Design review of the part built by this model. Coordinates are the model's own, in mm. A direction names the side the tool comes from. Coordinates: 2 decimals unless noted, no trailing zeros. Order: outer loops, then holes, each group sorted by start corner. A loop starts at its lowest first (then second) coordinate and runs counter-clockwise, first axis right, second up. Notation, with made-up numbers: (82.5, 78) -> (121.5, 78) arc R33 cw to (121.5, 108) -> close; hole circle Ø2 at (2.5, 51). An arc over 180 degrees is marked (long way). Use a Markdown table: item, result. Add a question column.
Q1. Add section C-C (x = -0.5). State the section outline as (y, z) points, then the cut area to 3 significant figures.
Q2. Wall thickness on probe 1 along X at (y, z) = (20, 1.1); probe 2 along X at (y, z) = (11.5, 0.85); probe 3 along X at (y, z) = (17, 5.6): over which ranges is each line inside the solid? List them lowest first.
Q3. Insertion check: pin 1 (3 mm diameter, centred on y = 14, z = 3, fed in from -X); pin 2 (1.8 mm diameter, centred on y = -2, z = 2, fed in from +X); pin 3 (0.9 mm diameter, centred on x = 11.5, z = 2.5, fed in from -Y). Each pin has a flat end and moves straight along its axis. Give the tip position at first contact, or say it passes through.
Q4. Machinability: for faces 1 (the face through (10, 15, 3)), 2 (the face through (7.21, 20.62, 3.04)), 3 (the face through (11, 0, 3)), 4 (the face through (-2, 0, 3)), 5 (the face through (13, 1, 3)), which of the approach directions +Z, -Z, +X, -X, +Y, -Y give a long, thin tool a straight path to every point of the face, cutting with its end or side? Answer none if there is none.
Q5. The part is to be moulded in two halves that separate along X. For faces 6 (the face through (4.96, 15.25, 3.04)), 7 (the face through (1, 25, 3)), 8 (the face through (0, 15, 3)), say which applies: pulls with the +X half, pulls with the -X half, needs draft (parallel to the pull), parting line crosses it, or undercut.
Q6. Add section B-B (y = -3). State the section outline as (x, z) points.
Autodesk Inventor part; units mm, degrees
ref_plane "YZ Plane" through (0, 0, 0) normal (1, 0, 0) x (0, 1, 0)
ref_plane "XZ Plane" through (0, 0, 0) normal (0, 1, 0) x (-1, 0, 0)
ref_plane "XY Plane" through (0, 0, 0) normal (0, 0, 1) x (1, 0, 0)
sketch "Sketch1" plane through (0, 0, 0) normal (0, 0, 1) x (1, 0, 0)
  line L0 (0, -6) -> (0, 0)
  line L1 (-9, 0) -> (0, 0)
  line L2 (0, -6) -> (-9, -6)
  line L3 (0, 0) -> (10, 0)
  line L4 (0, 0) -> (0, -6)
  line L5 (10, -6) -> (0, -6)
  line L6 (10, 0) -> (10, -6)
  line L7 (0, -6) -> (-9, -6)
  line L8 (-9, 0) -> (0, 0)
  line L9 (0, -6) -> (10, -6)
  line L10 (10, -6) -> (10, 0)
  line L11 (10, 0) -> (0, 0)
  line L12 (0, 0) -> (0, -6)
  line L13 (-3, 0) -> (13, 0)
  line L14 (13, 0) -> (13, 2)
  line L15 (13, 2) -> (-3, 2)
  line L16 (-3, 2) -> (-3, 0)
  line L17 (-9, -6) -> (-9, 0)
  line L18 (-9, -6) -> (-9, 0)
  line L19 (0, -6) -> (0, 0)
  point P0 (5, 2)
  point P1 (5, 0)
  dimension "d0" = 16
  dimension "d2" = 2
extrude "Extrusion1" add sketch "Sketch1" along normal blind 6 contours L0 L3 L6 L5 | L1 L16 L15 L14 L13 L3
sketch "Sketch2" plane through (0, 0, 6) normal (0, 0, 1) x (1, 0, 0)
  line L0 (0, 0) -> (0, -6)
  line L1 (0, -6) -> (10, -6)
  line L2 (10, -6) -> (10, 0)
  line L3 (13, 2) -> (-3, 2)
  line L4 (0, 2) -> (10, 2)
  line L5 (10, 2) -> (10, 25)
  line L6 (10, 25) -> (0, 25)
  line L7 (0, 25) -> (0, 2)
  dimension "d6" = 31
  dimension "d21" = 10
extrude "Extrusion2" add sketch "Sketch2" against normal blind 6
chamfer "Chamfer1" distance 3 angle 45 2 edges at (0, 2, 3) (10, 2, 3)
sketch "Sketch3" plane through (0, 0, 6) normal (0, 0, 1) x (1, 0, 0)
  line L0 (10, 5) -> (10, 25)
  line L1 (10, 25) -> (0, 25)
  line L2 (0, 25) -> (0, 5)
  line L3 (2.25, 25) -> (7.75, 25)
  line L4 (7.75, 25) -> (7.75, 17) construction
  line L5 (7.75, 17) -> (2.25, 17) construction
  line L6 (2.25, 17) -> (2.25, 25) construction
  circle A0 centre (5, 17) radius 1.75
  line L7 (-3, 0) -> (0, 0)
  line L8 (0, 0) -> (0, -6)
  line L9 (0, -6) -> (10, -6)
  line L10 (10, -6) -> (10, 0)
  line L11 (10, 0) -> (13, 0)
  line L12 (13, 0) -> (13, 2)
  line L13 (10, 5) -> (13, 2)
  line L14 (10, 5) -> (10, 25)
  line L15 (10, 25) -> (0, 25)
  line L16 (0, 25) -> (0, 5)
  line L17 (-3, 2) -> (0, 5)
  line L18 (-3, 2) -> (-3, 0)
  line L19 (6.7368, 16.7858) -> (7.75, 25)
  line L20 (2.25, 25) -> (3.2632, 16.7858)
  dimension "d12" = 2.25
  dimension "d13" = 2.25
  dimension "d14" = 8
  dimension "d17" = 3.5
extrude "Extrusion3" cut sketch "Sketch3" against normal blind 6 contours L19 A0 L20 L1 | A0
fillet "Fillet1" radius 0.5 4 edges at (7.75, 25, 3) (2.25, 25, 3) (0, 25, 3) (10, 25, 3)
properties part number "arm 1"
Established:
| question | item | result |
|---|---|---|
| 1 | outline | (0, 0) -> (4.5, 0) -> (4.5, 6) -> (0, 6) -> close |
| 1 | area | 27.0 mm^2 |
| 2 | probe 1 | 0 to 2.87, 7.13 to 10 |
| 2 | probe 2 | 0 to 10 |
| 2 | probe 3 | 0 to 3.24, 6.76 to 10 |
| 3 | pin 1 | x = 0 |
| 3 | pin 2 | x = 10 |
| 3 | pin 3 | y = 0 |
| 4 | face 1 | +Z, -Z, +X, +Y |
| 4 | face 2 | +Z, -Z, +Y |
| 4 | face 3 | +Z, -Z, +X, -Y |
| 4 | face 4 | +Z, -Z, -X, -Y |
| 4 | face 5 | +Z, -Z, +X, +Y, -Y |
| 5 | face 6 | undercut |
| 5 | face 7 | needs draft |
| 5 | face 8 | pulls with the -X half |
| 6 | outline | (0, 0) -> (10, 0) -> (10, 6) -> (0, 6) -> close |
